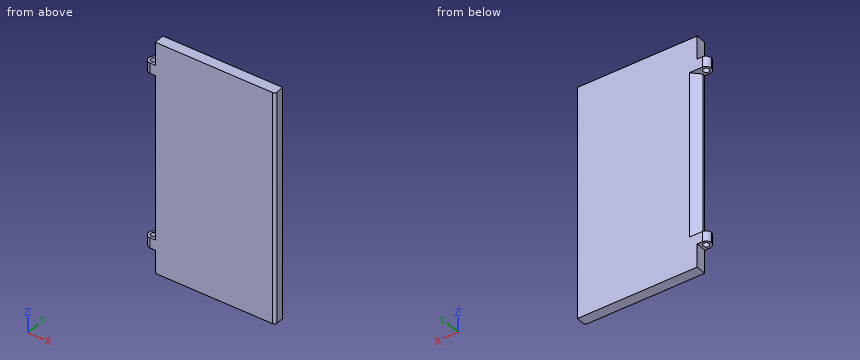
```python
from build123d import *

# Parameters (mm, degrees)
SKETCH_2_W             = 46
SKETCH_2_H             = 4
EXTRUDE_1_DEPTH        = 90
SKETCH_3_W             = 4
SKETCH_3_H             = 4
EXTRUDE_2_DEPTH        = 4
FILLET_1_R             = 2
CUT_EXTRUDE_1_REACH    = 91.783
SKETCH_4_R             = 1.15
FILLET_1_OF_MIRROR_3_R = 2
FILLET_2_R             = 1
CHAMFER_1_SIZE         = 3


with BuildPart() as part:
    # 草图2 → 凸台-拉伸1 (new body)
    with BuildSketch(Plane.XY):
        with Locations((23, 2)):
            Rectangle(SKETCH_2_W, SKETCH_2_H)
    extrude(amount=EXTRUDE_1_DEPTH)

    # 草图3 → 凸台-拉伸2 (add)
    with BuildSketch(Plane.ZY):
        with Locations((11, 2)):
            Rectangle(SKETCH_3_W, SKETCH_3_H)
    extrude_2 = extrude(amount=EXTRUDE_2_DEPTH)

    # 圆角1
    fillet_1_edges = [part.edges().sort_by_distance(p)[0] for p in [
        (-4, 4, 11),
        (-4, 0, 11),
    ]]
    fillet(fillet_1_edges, radius=FILLET_1_R - 0.0001)  # a hair under: the kernel refuses the full size

    # 草图4 → 切除-拉伸1 (cut, up to next)
    with BuildSketch(Plane.XY.offset(13), mode=Mode.PRIVATE) as cut_extrude_1_sk1:
        with Locations((-2, 2)):
            Circle(SKETCH_4_R)
    cut_extrude_1_tool1 = extrude(cut_extrude_1_sk1.sketch, amount=-CUT_EXTRUDE_1_REACH, mode=Mode.PRIVATE) & part.part
    cut_extrude_1 = cut_extrude_1_tool1.solids().sort_by_distance((-2, 2, 13))[0]
    add(cut_extrude_1, mode=Mode.SUBTRACT)

    # 镜向3: 凸台-拉伸2, 切除-拉伸1 across plane
    add(extrude_2.mirror(Plane(origin=(0, 0, 45), x_dir=(1, 0, 0), z_dir=(0, 0, -1))))
    add(cut_extrude_1.mirror(Plane(origin=(0, 0, 45), x_dir=(1, 0, 0), z_dir=(0, 0, -1))), mode=Mode.SUBTRACT)

    # 圆角1 of 镜向3
    fillet_1_of_mirror_3_edges = [part.edges().sort_by_distance(p)[0] for p in [
        (-4, 4, 79),
        (-4, 0, 79),
    ]]
    fillet(fillet_1_of_mirror_3_edges, radius=FILLET_1_OF_MIRROR_3_R - 0.0001)  # a hair under: the kernel refuses the full size

    # 圆角2
    fillet_2_edges = [part.edges().sort_by_distance(p)[0] for p in [
        (46, 0, 45),
    ]]
    fillet(fillet_2_edges, radius=FILLET_2_R)

    # 倒角1
    chamfer_1_edges = [part.edges().sort_by_distance(p)[0] for p in [
        (0, 4, 45),
    ]]
    chamfer(chamfer_1_edges, length=CHAMFER_1_SIZE)


solid = part.part
```
Check sheet for the modelled part. Datum: model origin and axes. Units: mm. Coordinates: 2 decimals unless noted, no trailing zeros. Order: outer loops, then holes, each group sorted by start corner. A loop starts at its lowest first (then second) coordinate and runs counter-clockwise, first axis right, second up. Notation, with made-up numbers: (73, 43.5) -> (110, 43.5) arc R9 cw to (110, 56.5) -> close; hole circle Ø8 at (39, -38). An arc over 180 degrees is marked (long way). Write item = value, one per line. Start each with the question number.
1) Material ranges on L1, parallel to Y at x = -2, z = 11.7; L2, parallel to X at y = 2, z = 43; L3, parallel to X at y = 1.5, z = 38.5, recorded low to high.
2) Go/stop test with flat-tipped pins: P1, Ø2, axis at x = -2, y = 2, coming from the -Z side; P2, Ø2, axis at y = 2.5, z = 2.5, coming from the -X side; P3, Ø1.2, axis at x = -2.5, y = 3, coming from the +Z side. Record where each tip stops, or that it passes through.
3) Cross-section at B-B (z = 59.5). Enter the section's corners in (x, y).
Ans:
q1.L1 = 0 to 0.85, 3.15 to 4
q1.L2 = 1 to 46
q1.L3 = 0.5 to 46
q2.P1 = through
q2.P2 = 0
q2.P3 = 81
q3.outline = (0, 0) -> (45, 0) arc R1 ccw to (46, 1) -> (46, 4) -> (3, 4) -> (0, 1) -> close
